Design review of the part built by this model. Coordinates are the model's own, in mm. Face numbers are marked on the shaded views. A direction names the side the tool comes from. Give positions to 0.01 mm unless a question says otherwise; leave off trailing zeros. Write each loop counter-clockwise with the first axis right and the second up, starting at its lowest first coordinate (ties: lowest second). Pieces come first, ordered by that corner, then holes. Notation, with made-up numbers: (-11, -24) -> (27, -24) arc R32 ccw to (27, 9) -> close; hole circle Ø4 at (44.25, 69). An arc over 180 degrees is marked (long way). Return JSON: item names as keys, results as strings. Group by question number.
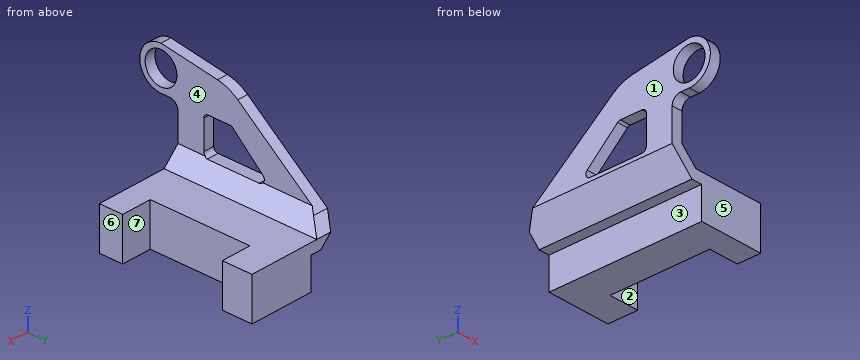
from build123d import *

# Parameters (mm, degrees)
SZKIC1_W                    = 15
SZKIC1_H                    = 36
DODANIE_WYCI_GNI_CIE1_DEPTH = 9.9
SZKIC2_W                    = 7
SZKIC2_H                    = 23.5
WYTNIJ_WYCI_GNI_CIE1_DEPTH  = 9.9
SZKIC3_R                    = 2.5
DODANIE_WYCI_GNI_CIE2_DEPTH = 7.5
WYTNIJ_WYCI_GNI_CIE2_DEPTH  = 137.5
WYTNIJ_WYCI_GNI_CIE3_DEPTH  = 137.5
ZAOKR_GLENIE1_R             = 10
ZAOKR_GLENIE2_R             = 2
SZKIC6_R                    = 3.75
WYTNIJ_WYCI_GNI_CIE4_DEPTH  = 10


with BuildPart() as part:
    # Szkic1 → Dodanie-wyciągnięcie1 (new body)
    with BuildSketch(Plane.XY):
        with Locations((-7.5, 18)):
            Rectangle(SZKIC1_W, SZKIC1_H)
    extrude(amount=DODANIE_WYCI_GNI_CIE1_DEPTH)

    # Szkic2 → Wytnij-wyciągnięcie1 (cut)
    with BuildSketch(Plane.XY.offset(9.9)):
        with Locations((-3.5, 17.25)):
            Rectangle(SZKIC2_W, SZKIC2_H)
    extrude(amount=-WYTNIJ_WYCI_GNI_CIE1_DEPTH, mode=Mode.SUBTRACT)

    # Szkic3 → Dodanie-wyciągnięcie2 (add)
    with BuildSketch(Plane.ZY.offset(15)):
        with BuildLine():
            Line((7.4, 36), (9.9, 36))
            Line((9.9, 36), (12.4, 32.923076923))
            Line((12.4, 32.923076923), (29.4, 12))
            Line((29.4, 12), (31.9, -4))
            ThreePointArc((31.9, -4), (26.9, -9), (21.9, -4))
            Line((21.9, -4), (21.9, 0))
            Line((21.9, 0), (12.4, 0))
            Line((12.4, 0), (7.4, 0))
            Line((7.4, 0), (7.4, 36))
        make_face()
        with Locations((26.9, -4)):
            Circle(SZKIC3_R, mode=Mode.SUBTRACT)
    extrude(amount=DODANIE_WYCI_GNI_CIE2_DEPTH)

    # Szkic4 → Wytnij-wyciągnięcie2 (cut)
    with BuildSketch(Plane(origin=(0, 36, 0), x_dir=(1, 0, 0), z_dir=(0, 1, 0))):
        Polygon((-17.5, -7.4), (-25.001097051, -14.901097051), (-26.525986736, -7.4), align=None)
        Polygon((-16.464466094, -9.9), (-20, -13.435533906), (-20, -34.97095788), (-2.856589665, -34.97095788), (-4.384348652, -9.9), align=None)
    extrude(amount=-WYTNIJ_WYCI_GNI_CIE2_DEPTH, mode=Mode.SUBTRACT)

    # Szkic5 → Wytnij-wyciągnięcie3 (cut)
    with BuildSketch(Plane.ZY.offset(22.5)):
        with BuildLine():
            Line((14.930271414, 20.050399523), (21.630271414, 12.888330558))
            ThreePointArc((21.630271414, 12.888330558), (21.830126715, 12.572412171), (21.9, 12.205173429))
            Line((21.9, 12.205173429), (21.9, 7.1))
            ThreePointArc((21.9, 7.1), (21.607106781, 6.392893219), (20.9, 6.1))
            Line((20.9, 6.1), (14.2, 6.1))
            ThreePointArc((14.2, 6.1), (13.492893219, 6.392893219), (13.2, 7.1))
            Line((13.2, 7.1), (13.2, 19.367242395))
            ThreePointArc((13.2, 19.367242395), (13.832761259, 20.29736911), (14.930271414, 20.050399523))
        make_face()
    extrude(amount=-WYTNIJ_WYCI_GNI_CIE3_DEPTH, mode=Mode.SUBTRACT)

    # Zaokrąglenie1
    zaokr_glenie1_edges = [part.edges().sort_by_distance(p)[0] for p in [
        (-21.25, 12, 29.4),
    ]]
    fillet(zaokr_glenie1_edges, radius=ZAOKR_GLENIE1_R)

    # Zaokrąglenie2
    zaokr_glenie2_edges = [part.edges().sort_by_distance(p)[0] for p in [
        (-21.25, 0, 21.9),
    ]]
    fillet(zaokr_glenie2_edges, radius=ZAOKR_GLENIE2_R)

    # Szkic6 → Wytnij-wyciągnięcie4 (cut)
    with BuildSketch(Plane.ZY.offset(22.5)):
        with Locations((26.9, -4)):
            Circle(SZKIC6_R)
    extrude(amount=-WYTNIJ_WYCI_GNI_CIE4_DEPTH, mode=Mode.SUBTRACT)


solid = part.part
Q1. Insertion check: pin 1 (5 mm diameter, centred on y = 0.5, z = 24, fed in from +X); pin 2 (3.5 mm diameter, centred on x = -2, z = 3.5, fed in from -Y); pin 3 (3 mm diameter, centred on x = -12, y = 22, fed in from +Z). Each pin has a flat end and moves straight along its axis. Give the tip position at first contact, or say it passes through.
Q2. Take a section at D-D, the plane z = 26.9. Give the boundary of the cut face in (x, y), plus the area to 3 significant figures.
Q3. Take a section at A-A, the plane x = -1.75. Give the boundary of the cut face in (y, z), plus the area to 3 significant figures.
Q4. Take a section at C-C, the plane y = 28. Give the boundary of the cut face in (x, z), plus the area to 3 significant figures.
Q5. For L1, parallel to Y at x = -1.5, z = 9; L2, parallel to Z at x = -8.75, y = 5.5; L3, parallel to Y at x = -21.35, z = 26.9, list the stretches that pass through material, from the lowest coordinate up. Write a range as from..to.
Q6. Take a section at B-B, the plane y = 16. Give the boundary of the cut face in (x, z).
Q7. Tool access review of the marked faces 1, 2, 3 and 4: name each direction out of +Z, -Z, +X, -X, +Y, -Y from which nothing blocks a thin tool from reaching the whole face with its end or side.
Q8. Mouldability with a two-part tool opening along Y and no side actions: class the marked faces 5, 6 and 7 as +Y half, -Y half, draft (parallel to the pull), parting line (faces both ways), or undercut.
Final values:
{
 "1": {"pin 1": "stops at x = -20", "pin 2": "stops at y = 0", "pin 3": "stops at z = 9.9"},
 "2": {"outline": "(-22.5, -9) -> (-20, -9) -> (-20, -7.75) -> (-22.5, -7.75) -> close; (-22.5, -0.25) -> (-20, -0.25) -> (-20, 15.08) -> (-22.5, 15.08) -> close", "area": "41.4 mm²"},
 "3": {"outline": "(0, 0) -> (5.5, 0) -> (5.5, 9.9) -> (0, 9.9) -> close; (29, 0) -> (36, 0) -> (36, 9.9) -> (29, 9.9) -> close", "area": "124 mm²"},
 "4": {"outline": "(-22.5, 12.4) -> (-17.5, 7.4) -> (-15, 7.4) -> (-15, 0) -> (-7, 0) -> (-7, 9.9) -> (-16.46, 9.9) -> (-20, 13.44) -> (-20, 16.4) -> (-22.5, 16.4) -> close", "area": "108 mm²"},
 "5": {"L1": "y = 0..5.5, 29..36", "L2": "z = 0..9.9", "L3": "y = -9..-7.75, -0.25..15.08"},
 "6": {"outline": "(-22.5, 12.4) -> (-17.5, 7.4) -> (-15, 7.4) -> (-15, 0) -> (-7, 0) -> (-7, 9.9) -> (-16.46, 9.9) -> (-19.76, 13.2) -> (-22.5, 13.2) -> close; (-22.5, 18.72) -> (-20, 18.72) -> (-20, 26.15) -> (-22.5, 26.15) -> close"},
 "7": {"face 1": "+Z, -Z, -X, +Y, -Y", "face 2": "+Z, -Z, +X", "face 3": "-Z, -X, +Y, -Y", "face 4": "+Z, +X, +Y, -Y"},
 "8": {"face 5": "-Y half", "face 6": "draft", "face 7": "undercut"}
}
